```python
from build123d import *

# Parameters (mm, degrees)
F0_R     = 3.95
F0_R_2   = 2.54
F0_R_3   = 1
F1_DEPTH = 1.5
F2_DEPTH = 8.2
F3_DEPTH = 9.5


with BuildPart() as f1:
    # F0 (on Top) → F1 (new body)
    with BuildSketch(Plane.XY):
        with BuildLine():
            Line((2.319022, -18.354077), (0, -16))
            ThreePointArc((0, -16), (-1.348069, -15.943109), (-2.686551, -15.772839))
            Line((-2.686551, -15.772839), (0, -18.5))
            ThreePointArc((0, -18.5), (1.161804, -18.463483), (2.319022, -18.354077))
        make_face()
        with BuildLine():
            ThreePointArc((0, -18.5), (-9.231437, -16.032173), (-16, -9.287088))
            Line((-16, -9.287088), (-16, -23.633545))
            Line((-16, -23.633545), (0, -23.633545))
            Line((0, -23.633545), (0, -20.048685))
            Line((0, -20.048685), (0, -18.5))
        make_face()
        with BuildLine():
            ThreePointArc((-2.686551, -15.772839), (-12.226709, -10.320251), (-16, 0))
            Line((-16, 0), (-16, -9.287088))
            ThreePointArc((-16, -9.287088), (-9.231437, -16.032173), (0, -18.5))
            Line((0, -18.5), (-2.686551, -15.772839))
        make_face()
        with BuildLine():
            ThreePointArc((0, -16), (11.313708, -11.313708), (16, 0))
            ThreePointArc((16, 0), (0, 16), (-16, 0))
            ThreePointArc((-16, 0), (-12.226709, -10.320251), (-2.686551, -15.772839))
            ThreePointArc((-2.686551, -15.772839), (-1.348069, -15.943109), (0, -16))
        make_face()
        Circle(F0_R, mode=Mode.SUBTRACT)
        Circle(F0_R)
        Circle(F0_R_2, mode=Mode.SUBTRACT)
        with BuildLine():
            ThreePointArc((-16, 0), (0, 16), (16, 0))
            ThreePointArc((16, 0), (11.313708, -11.313708), (0, -16))
            Line((0, -16), (2.319022, -18.354077))
            ThreePointArc((2.319022, -18.354077), (13.877174, -12.234134), (18.5, 0))
            ThreePointArc((18.5, 0), (0, 18.5), (-18.5, 0))
            Line((-18.5, 0), (-16, 0))
        make_face()
        with Locations((0, 17.25)):
            Circle(F0_R_3, mode=Mode.SUBTRACT)
        with BuildLine():
            Line((-16, -9.287088), (-16, 0))
            Line((-16, 0), (-18.5, 0))
            ThreePointArc((-18.5, 0), (-17.86407, -4.808846), (-16, -9.287088))
        make_face()
        with BuildLine():
            Line((-16, -23.633545), (-16, -9.287088))
            ThreePointArc((-16, -9.287088), (-17.86407, -4.808846), (-18.5, 0))
            Line((-18.5, 0), (-18.5, -23.633545))
            Line((-18.5, -23.633545), (-16, -23.633545))
        make_face()
        with BuildLine():
            Line((2.319022, -23.633545), (2.319022, -18.354077))
            ThreePointArc((2.319022, -18.354077), (1.161804, -18.463483), (0, -18.5))
            Line((0, -18.5), (0, -20.048685))
            Line((0, -20.048685), (0, -23.633545))
            Line((0, -23.633545), (2.319022, -23.633545))
        make_face()
    extrude(amount=-F1_DEPTH)

    # F0 (on Top) → F2 (join)
    with BuildSketch(Plane.XY):
        with BuildLine():
            Line((-16, -23.633545), (-16, -9.287088))
            ThreePointArc((-16, -9.287088), (-17.86407, -4.808846), (-18.5, 0))
            Line((-18.5, 0), (-18.5, -23.633545))
            Line((-18.5, -23.633545), (-16, -23.633545))
        make_face()
        with BuildLine():
            Line((-16, -9.287088), (-16, 0))
            Line((-16, 0), (-18.5, 0))
            ThreePointArc((-18.5, 0), (-17.86407, -4.808846), (-16, -9.287088))
        make_face()
        with BuildLine():
            ThreePointArc((-16, 0), (0, 16), (16, 0))
            ThreePointArc((16, 0), (11.313708, -11.313708), (0, -16))
            Line((0, -16), (2.319022, -18.354077))
            ThreePointArc((2.319022, -18.354077), (13.877174, -12.234134), (18.5, 0))
            ThreePointArc((18.5, 0), (0, 18.5), (-18.5, 0))
            Line((-18.5, 0), (-16, 0))
        make_face()
        with Locations((0, 17.25)):
            Circle(F0_R_3, mode=Mode.SUBTRACT)
        with BuildLine():
            Line((2.319022, -23.633545), (2.319022, -18.354077))
            ThreePointArc((2.319022, -18.354077), (1.161804, -18.463483), (0, -18.5))
            Line((0, -18.5), (0, -20.048685))
            Line((0, -20.048685), (0, -23.633545))
            Line((0, -23.633545), (2.319022, -23.633545))
        make_face()
        with BuildLine():
            Line((2.319022, -18.354077), (0, -16))
            ThreePointArc((0, -16), (-1.348069, -15.943109), (-2.686551, -15.772839))
            Line((-2.686551, -15.772839), (0, -18.5))
            ThreePointArc((0, -18.5), (1.161804, -18.463483), (2.319022, -18.354077))
        make_face()
        Circle(F0_R)
        Circle(F0_R_2, mode=Mode.SUBTRACT)
    extrude(amount=F2_DEPTH)

    # F0 (on Top) → F3 (join)
    with BuildSketch(Plane.XY):
        with Locations((0, 17.25)):
            Circle(F0_R_3)
        Circle(F0_R_2)
    extrude(amount=F3_DEPTH)


solid = f1.part
```
Could you check a few things on this model? Use its own coordinates, in mm. A direction names the side the tool comes from. Round coordinates to 2 decimals unless told otherwise and drop trailing zeros. Write each loop counter-clockwise with the first axis right and the second up, starting at its lowest first coordinate (ties: lowest second). Pieces come first, ordered by that corner, then holes. Notation, with made-up numbers: M 22.25,78 L 69.25,78 A17 ccw 69.25,104 Z; hole C 78.25,-39 d4. An arc over 180 degrees is marked long. Answer in a Markdown table with one row per item. Add a question column.
Q1. Imagine slicing it at B-B (y = 11). Please give me the cut outline in (x, z), then the cut area to 3 significant figures.
Q2. If I drill on line 1 (Y direction, x = 0, z = -0.5); line 2 (X direction, y = -2.5, z = 3); line 3 (Z direction, x = 10, y = -15.5), over which ranges is the centre line in solid material (lowest first)? Write a range as from..to.
Q3. Imagine slicing it at C-C (x = 6). Please give me the cut outline in (y, z), then the cut area to 3 significant figures.
Q4. Imagine slicing it at D-D (x = -7). Please give me the cut outline in (y, z).
Q5. If we mould it in two halves opening along X, with no side actions, what happens to faces 5 (the flat face through (0, 17, 0)), 6 (the cylindrical face through (-0.217, 16.274, 8.841)), 7 (the flat face through (0, 0, 9.5)), 8 (the flat face through (-18.5, -12, 3))? For each: +X half, -X half, draft (parallel to the pull), parting line (faces both ways), or undercut.
Q6. Imagine slicing it at A-A (z = 2.5). Please give me the cut outline in (x, y), then the cut area to 3 significant figures.
Q7. On a 3-axis mill with a long thin cutter (end or side, diameter ignored), from which of +Z, -Z, +X, -X, +Y, -Y can I reach the whole of each face in a straight line? I mean faces 1 (the cylindrical face through (-0.33, 2.52, -0.74)), 2 (the flat face through (2.319, -21, 3)), 3 (the flat face through (-1.36, -17.12, 4.04)), 4 (the cylindrical face through (-0.33, 2.52, 8.84)). Say none if no direction works.
Q8. Will these pins go through, and if not, where does the flat tip stop? pin 1 Ø6.5 at (y, z) = (-6.5, 4) entering from +X; pin 2 Ø5 at (x, z) = (-11.5, 7) entering from -Y; pin 3 Ø4 at (y, z) = (-22, 5) entering from +X.
Values:
| question | item | result |
|---|---|---|
| 1 | outline | M -14.87,-1.5 L 14.87,-1.5 L 14.87,8.2 L 11.62,8.2 L 11.62,0 L -11.62,0 L -11.62,8.2 L -14.87,8.2 Z |
| 1 | area | 98.0 mm^2 |
| 2 | line 1 | -23.63..-2.54, 2.54..16.25, 18.25..18.5 |
| 2 | line 2 | -18.5..-16, -3.06..3.06, 15.8..18.33 |
| 2 | line 3 | -1.5..8.2 |
| 3 | outline | M -17.5,-1.5 L 17.5,-1.5 L 17.5,8.2 L 14.83,8.2 L 14.83,0 L -14.83,0 L -14.83,8.2 L -17.5,8.2 Z |
| 3 | area | 96.2 mm^2 |
| 4 | outline | M -23.63,-1.5 L 17.12,-1.5 L 17.12,8.2 L 14.39,8.2 L 14.39,0 L -23.63,0 Z |
| 5 | face 5 | undercut |
| 5 | face 6 | parting line |
| 5 | face 7 | draft |
| 5 | face 8 | -X half |
| 6 | outline | M -18.5,-23.63 L -16,-23.63 L -16,0 A16 cw 16,0 A16 cw 0,-16 A16 cw -2.69,-15.77 L 0,-18.5 L 0,-23.63 L 2.32,-23.63 L 2.32,-18.35 A18.5 ccw long -18.5,0 Z; C 0,0 d7.9 |
| 6 | area | 327 mm^2 |
| 7 | face 1 | -Z |
| 7 | face 2 | +Z, -Z, +X, -Y |
| 7 | face 3 | +Z, -Y |
| 7 | face 4 | +Z |
| 8 | pin 1 | x = 18.21 |
| 8 | pin 2 | y = 7.75 |
| 8 | pin 3 | x = 2.32 |
